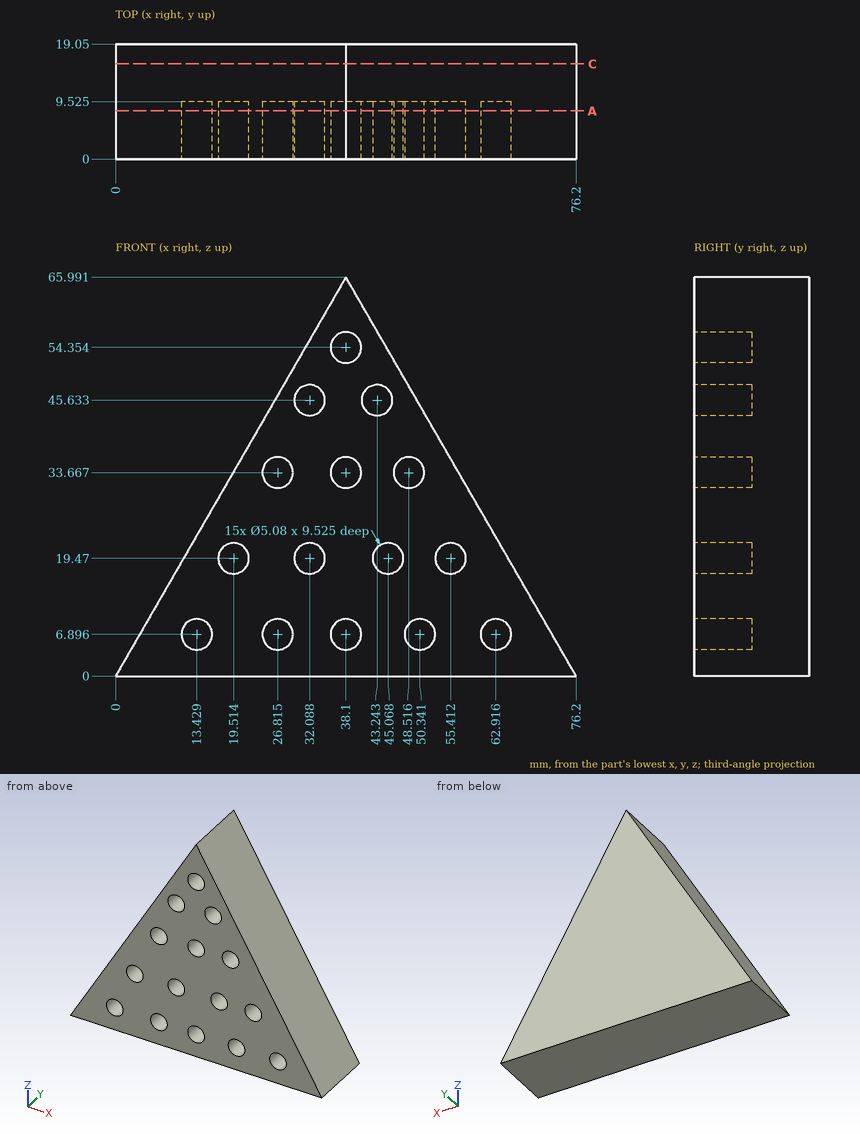
Design review of the part shown in the three views and the two pictorial views. Dimensions are in mm from the part's minimum x, y and z. Round coordinates to 2 decimals unless told otherwise and drop trailing zeros. Loops run counter-clockwise (first coordinate to the right, second up) from the corner with the lowest first, then second, coordinate; pieces in that order, holes last. Notation, with made-up numbers: (31.5, 17) -> (57.5, 17) arc R21 cw to (57.5, 24) -> close; hole circle Ø1 at (89, 6). An arc over 180 degrees is marked (long way). Answer as a JSON object with one key per item and string values. Group by question number.
1) For pin 1 Ø2.5 at (x, z) = (51, 6) entering from -Y (3 decimals); pin 2 Ø1.5 at (y, z) = (16.5, 17.5) entering from +X; pin 3 Ø1 at (y, z) = (12.5, 49.5) entering from -X, all flat-tipped, find the tip position at first contact; note any pin that passes through.
2) We need section A-A on y = 8. Give the number of separate pieces and of enclosed holes in the cut face, then the cut area to 3 significant figures.
3) For line 1 (Z direction, x = 32, y = 3.5) (1 decimal); line 2 (X direction, y = 6.5, z = 18.5) (1 decimal); line 3 (Z direction, x = 63.5, y = 5) (1 decimal), list the stretches that pass through material, from the lowest coordinate up. Write a range as [from, to].
4) We need section C-C on y = 15.75. Write out the cut boundary in (x, z), then the cut area to 3 significant figures.
Result set:
{
 "1": {"pin 1": "y = 9.525", "pin 2": "x = 66.53", "pin 3": "x = 28.29"},
 "2": {"separate pieces": "1", "enclosed holes": "15", "area": "2,210 mm²"},
 "3": {"line 1": "[0, 16.9], [22, 43.1], [48.2, 55.4]", "line 2": "[10.7, 17.2], [21.9, 29.7], [34.4, 42.7], [47.4, 53.1], [57.8, 65.5]", "line 3": "[0, 4.4], [9.4, 22]"},
 "4": {"outline": "(0, 0) -> (76.2, 0) -> (38.1, 65.99) -> close", "area": "2,510 mm²"}
}
